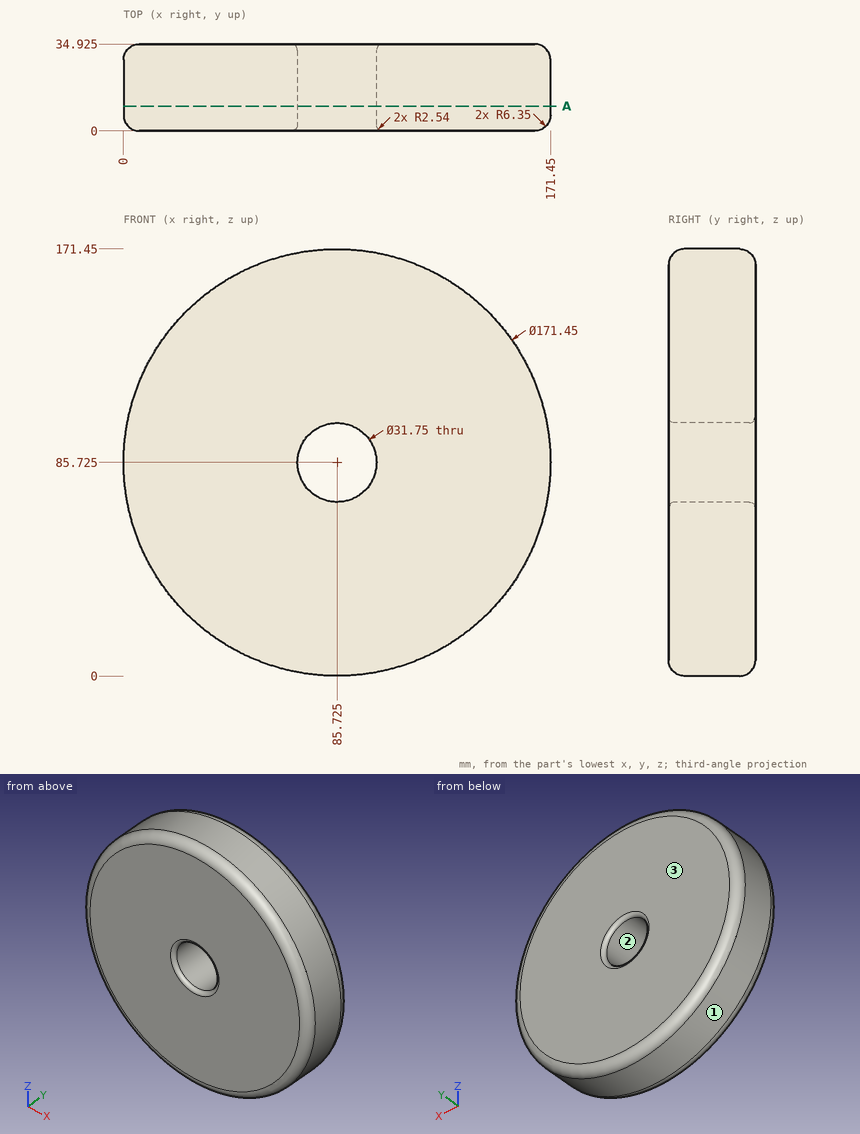
Could you check a few things on this drawing? It's one solid part, dimensions in mm from its lowest x, y, z. Coordinates: 2 decimals unless noted, no trailing zeros. Order: outer loops, then holes, each group sorted by start corner. A loop starts at its lowest first (then second) coordinate and runs counter-clockwise, first axis right, second up.
1. If we section it at A-A (y = 10): Please give me the cut outline in (x, z) (3 decimals).
2. I need wall thicknesses on line 1 (Z direction, x = 73, y = 33.5); line 2 (X direction, y = 25, z = 154); line 3 (Z direction, x = 65, y = 9.5). Which ranges of each line are inside material? Lowest first, please.
3. Thinking about a two-plate mould opening in X: for the marked faces 1, 2 and 3, which applies, +X half, -X half, draft (parallel to the pull), parting line (faces both ways), or undercut?
4. I'm going to push flat-ended pins straight in: pin 1 (1 mm diameter, centred on x = 17, y = 17, fed in from -Z); pin 2 (2 mm diameter, centred on y = 7, z = 149, fed in from -X); pin 3 (5 mm diameter, centred on y = 23.5, z = 36.5, fed in from -X). Where does each tip first touch, or does it pass through?
Entries:
1. outline: circle Ø171.45 at (85.725, 85.725); hole circle Ø31.75 at (85.725, 85.725)
2. line 1: z = 3.32 to 75.81, 95.64 to 168.13
2. line 2: x = 33.89 to 137.56
2. line 3: z = 2.54 to 168.91
3. face 1: parting line
3. face 2: undercut
3. face 3: draft
4. pin 1: stops at z = 33.82
4. pin 2: stops at x = 26.81
4. pin 3: stops at x = 13.85
